Part print with two shaded views. Sizes in mm from the minimum x, y, z corner. A direction names the side the tool comes from. Coordinates: 2 decimals unless noted, no trailing zeros. Loops run counter-clockwise (first coordinate to the right, second up) from the corner with the lowest first, then second, coordinate; pieces in that order, holes last.
(1) Slice it at D-D (y = 41). Give the cut face in (x, z), and give its area (3 significant figures).
(2) Two-plate mould, pull along X, no slides. Class the marked faces 1, 2, 3 and 4: pulls with the +X half, pulls with the -X half, needs draft (parallel to the pull), parting line crosses it, or undercut.
(3) Flat gauge pins, fed straight in: P1, Ø10, axis at y = 29.5, z = 34.5, coming from the -X side; P2, Ø5, axis at x = 92, y = 11, coming from the +Z side. Where does each tip first touch, or does it go through?
(4) Slice it at C-C (z = 10). Give the cut face in (x, y).
(5) Tool access for the marked faces 5 and 6: list every direction of +Z, -Z, +X, -X, +Y, -Y with a clear straight run to the whole face (end or side of a thin tool).
(6) Slice it at B-B (x = 120). Give the cut face in (y, z).
(7) Slice it at A-A (z = 24). Give the cut face in (x, y), and give its area (3 significant figures).
(8) Wall check: L1, parallel to Y at x = 77, z = 20; L2, parallel to Z at x = 120, y = 58.3; L3, parallel to X at y = 49.5, z = 24. Give the ranges that are in metal, low to high.
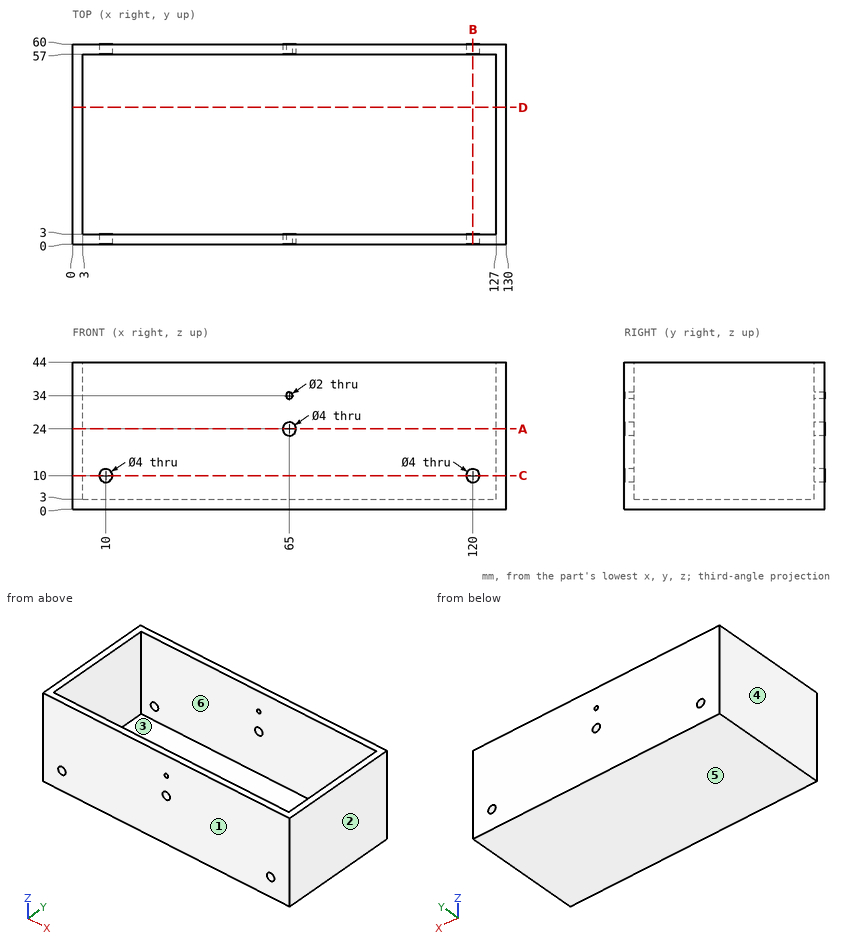
Response values:
1. outline: (0, 0) - (130, 0) - (130, 44) - (127, 44) - (127, 3) - (3, 3) - (3, 44) - (0, 44) - close
1. area: 636 mm2
2. face 1: needs draft
2. face 2: pulls with the +X half
2. face 3: undercut
2. face 4: pulls with the -X half
3. P1: stops at x = 0
3. P2: stops at z = 3
4. outline: (0, 0) - (8, 0) - (8, 3) - (3, 3) - (3, 57) - (8, 57) - (8, 60) - (0, 60) - close; (12, 0) - (118, 0) - (118, 3) - (12, 3) - close; (12, 57) - (118, 57) - (118, 60) - (12, 60) - close; (122, 0) - (130, 0) - (130, 60) - (122, 60) - (122, 57) - (127, 57) - (127, 3) - (122, 3) - close
5. face 5: -Z, +X, -X, +Y, -Y
5. face 6: +Z
6. outline: (0, 0) - (60, 0) - (60, 8) - (57, 8) - (57, 3) - (3, 3) - (3, 8) - (0, 8) - close; (0, 12) - (3, 12) - (3, 44) - (0, 44) - close; (57, 12) - (60, 12) - (60, 44) - (57, 44) - close
7. outline: (0, 0) - (63, 0) - (63, 3) - (3, 3) - (3, 57) - (63, 57) - (63, 60) - (0, 60) - close; (67, 0) - (130, 0) - (130, 60) - (67, 60) - (67, 57) - (127, 57) - (127, 3) - (67, 3) - close
7. area: 1,080 mm2
8. L1: y = 0 to 3, 57 to 60
8. L2: z = 0 to 8, 12 to 44
8. L3: x = 0 to 3, 127 to 130
